```python
from build123d import *

# Parameters (mm, degrees)
CROQUIS1_R              = 5
SALIENTE_EXTRUIR1_DEPTH = 12
CROQUIS2_R              = 4
CORTAR_EXTRUIR1_DEPTH   = 21
CROQUIS3_W              = 60
CROQUIS3_H              = 34
CORTAR_EXTRUIR4_DEPTH   = 1
CROQUIS5_R              = 3.2
CORTAR_EXTRUIR5_DEPTH   = 90.423598675


with BuildPart() as part:
    # Croquis1 → Saliente-Extruir1 (new body)
    with BuildSketch(Plane.XY):
        with BuildLine():
            Line((0, 12.7), (75, 12.7))
            ThreePointArc((75, 12.7), (87.7, 0), (75, -12.7))
            Line((75, -12.7), (0, -12.7))
            ThreePointArc((0, -12.7), (-12.7, 0), (0, 12.7))
        make_face()
        Circle(CROQUIS1_R, mode=Mode.SUBTRACT)
        with Locations((75, 0)):
            Circle(CROQUIS1_R, mode=Mode.SUBTRACT)
    extrude(amount=SALIENTE_EXTRUIR1_DEPTH)

    # Croquis2 → Cortar-Extruir1 (cut)
    with BuildSketch(Plane.XZ.offset(12.7)):
        with Locations(Location((37.5, 6, 0), (0, 0, 270))):
            Circle(CROQUIS2_R)
    extrude(amount=-CORTAR_EXTRUIR1_DEPTH, mode=Mode.SUBTRACT)

    # Croquis3 → Cortar-Extruir4 (cut)
    with BuildSketch(Plane.XY.offset(12)):
        with Locations((37.5, 0)):
            Rectangle(CROQUIS3_W, CROQUIS3_H)
    extrude(amount=-CORTAR_EXTRUIR4_DEPTH, mode=Mode.SUBTRACT)

    # Croquis5 → Cortar-Extruir5 (cut, through all)
    with BuildSketch(Plane.XY.offset(12)):
        with Locations((59.5, -6.7)):
            Circle(CROQUIS5_R)
        with Locations((59.5, 6.7)):
            Circle(CROQUIS5_R)
        with Locations((15.5, 6.7)):
            Circle(CROQUIS5_R)
        with Locations((15.5, -6.7)):
            Circle(CROQUIS5_R)
    extrude(amount=-CORTAR_EXTRUIR5_DEPTH, mode=Mode.SUBTRACT)


solid = part.part
```
Geometry check sheet. Reference: the model listing, model coordinates, mm. A direction names the side the tool comes from. Coordinates: 2 decimals unless noted, no trailing zeros. Write each loop counter-clockwise with the first axis right and the second up, starting at its lowest first coordinate (ties: lowest second). Pieces come first, ordered by that corner, then holes. Notation, with made-up numbers: M -11,51.5 L 20,51.5 A27 ccw 20,82.5 Z; hole C 3,1 d6. An arc over 180 degrees is marked long. Use one line per item in the form item = value. Start each with the question number.
1) Set-up check for faces 4 (the cylindrical face through (12.3, 6.8, 5.6)), 5 (the cylindrical face through (41.466, -2.347, 6.521)): record each of +Z, -Z, +X, -X, +Y, -Y from which the full face is reachable in a straight line by a thin tool's end or side.
2) Section check A-A on y = 0. Enter the section's corners in (x, z), and give its area (3 significant figures).
3) Section check C-C on x = 1.5. Enter the section's corners in (y, z), and give its area (3 significant figures).
4) Go/stop test with flat-tipped pins: pin 1 Ø7.5 at (x, y) = (38.5, 3) entering from +Z; pin 2 Ø2 at (y, z) = (-8, 7.5) entering from -X; pin 3 Ø2 at (y, z) = (-7.5, 7) entering from -X. Record where each tip stops, or that it passes through.
5) Release check for a two-part mould opening along Z. For faces 1 (the flat face through (38, -12.7, 1)), 2 (the flat face through (37, 0, 11)), 3 (the flat face through (38, 8.3, 6)) record: pulls with the +Z half, pulls with the -Z half, needs draft (parallel to the pull), parting line crosses it, or undercut.
6) Thickness scan on probe 1 along Y at (x, z) = (59.5, 4.5); probe 2 along X at (y, z) = (-8, 2.75); probe 3 along X at (y, z) = (-1, 7.25). Record the ranges inside material, lowest first. Write a range as from..to.
7) Section check B-B on x = 59.5. Enter the section's corners in (y, z), and give its area (3 significant figures).
8) Section check D-D on z = 3.5. Enter the section's corners in (x, y), and give its area (3 significant figures).
Responses:
q1.face_4 = +Z, -Z
q1.face_5 = -Y
q2.outline = M -12.7,0 L -5,0 L -5,12 L -12.7,12 Z; M 5,0 L 70,0 L 70,12 L 67.5,12 L 67.5,11 L 7.5,11 L 7.5,12 L 5,12 Z; M 80,0 L 87.7,0 L 87.7,12 L 80,12 Z; hole C 37.5,6 d8
q2.area = 855 mm2
q3.outline = M -12.7,0 L -4.77,0 L -4.77,12 L -12.7,12 Z; M 4.77,0 L 12.7,0 L 12.7,12 L 4.77,12 Z
q3.area = 190 mm2
q4.pin_1 = 11
q4.pin_2 = -10.6
q4.pin_3 = -10.91
q5.face_1 = needs draft
q5.face_2 = pulls with the +Z half
q5.face_3 = undercut
q6.probe_1 = -12.7..-9.9, -3.5..3.5, 9.9..12.7
q6.probe_2 = -9.86..12.58, 18.42..35.17, 39.83..56.58, 62.42..84.86
q6.probe_3 = -12.66..-4.9, 4.9..33.7, 41.3..70.1, 79.9..87.66
q7.outline = M -12.7,0 L -9.9,0 L -9.9,11 L -12.7,11 Z; M -3.5,0 L 3.5,0 L 3.5,11 L -3.5,11 Z; M 9.9,0 L 12.7,0 L 12.7,11 L 9.9,11 Z
q7.area = 139 mm2
q8.outline = M 0,-12.7 L 34.38,-12.7 L 34.38,8.3 L 40.62,8.3 L 40.62,-12.7 L 75,-12.7 A12.7 ccw 75,12.7 L 0,12.7 A12.7 ccw Z; hole C 0,0 d10; hole C 15.5,-6.7 d6.4; hole C 15.5,6.7 d6.4; hole C 59.5,-6.7 d6.4; hole C 59.5,6.7 d6.4; hole C 75,0 d10
q8.area = 1,990 mm2
